Autodesk Inventor part; units mm, degrees
ref_plane "YZ Plane" through (0, 0, 0) normal (1, 0, 0) x (0, 1, 0)
ref_plane "XZ Plane" through (0, 0, 0) normal (0, 1, 0) x (-1, 0, 0)
ref_plane "XY Plane" through (0, 0, 0) normal (0, 0, 1) x (1, 0, 0)
sketch "Sketch1" plane through (0, 0, 0) normal (1, 0, 0) x (0, 1, 0)
  line L0 (0, -12) -> (3, -12)
  line L1 (3, 12) -> (0, 12)
  line L2 (0, 12) -> (0, -12)
  line L3 (3, 9) -> (3, -9)
  line L4 (3, 0) -> (0, 0)
  line L5 (0, -9.75) -> (0, 9.75)
  line L6 (3, 9.75) -> (3, -9.75)
  line L7 (3, 10.75) -> (2.15, 10.75)
  line L8 (2.15, 10.75) -> (2.15, 9.75)
  line L9 (3, 12) -> (3, 10.75)
  line L10 (2.15, 9.75) -> (3, 9.75)
  line L11 (3, -10.75) -> (2.15, -10.75)
  line L12 (2.15, -10.75) -> (2.15, -9.75)
  line L13 (2.15, -9.75) -> (3, -9.75)
  line L14 (3, -10.75) -> (3, -12)
  line L15 (0, -16.8) -> (0, 16.8)
  point P0 (1.5, 0)
  dimension "d12" = 19.5
  dimension "d13" = 1
  dimension "d14" = 0.85
  dimension "d16" = 1
revolve "Revolution1" add sketch "Sketch1" angle 360 about axis through (0, 0, -10) along (0, 0, 1)
sketch "Sketch2" plane through (0, 0, 12) normal (0, 0, 1) x (1, 0, 0)
  circle A0 centre (0, 0) radius 3
extrude "Extrusion1" cut sketch "Sketch2" against normal blind 0.25
sketch "Sketch3" plane through (0, 0, -12) normal (0, 0, -1) x (-1, 0, 0)
  circle A0 centre (0, 0) radius 3
extrude "Extrusion2" cut sketch "Sketch3" against normal blind 0.25
chamfer "Chamfer1" distance 0.5 angle 45 2 edges at (0, -3, -11.75) (0, -3, 11.75)
properties part number "hridelka1"
Part model, mm, in its own coordinate system. A direction names the side the tool comes from. Give positions to 0.01 mm unless a question says otherwise; leave off trailing zeros. Write each loop counter-clockwise with the first axis right and the second up, starting at its lowest first coordinate (ties: lowest second). Pieces come first, ordered by that corner, then holes. Notation, with made-up numbers: (-10.5, 61.5) -> (35.5, 61.5) arc R24 cw to (35.5, 81.5) -> close; hole circle Ø10 at (13.25, -37). An arc over 180 degrees is marked (long way). Put each result on its own line as item: value. Start each with the question number.
Item 1: Cut at C-C (z = 6.5). List the corners of the cut face in (x, y), then the cut area to 3 significant figures.
Item 2: Pin check, flat tips, straight feed: pin 1 Ø2 at (x, z) = (1.5, 5) entering from -Y; pin 2 Ø1.5 at (y, z) = (-2, -6.5) entering from -X; pin 3 Ø1 at (y, z) = (1.5, 4) entering from +X. Stop position of each tip, or through.
Item 3: Which spindle directions (+Z, -Z, +X, -X, +Y, -Y) get a long thin tool onto all of the face, cutting with end or side? Do faces 1 (the face through (2, 1.3, -9.75)), 2 (the face through (0, -3, -11)). Say none if no direction does.
Item 4: Cut at A-A (y = 0). List the corners of the cut face in (x, z), then the cut area to 3 significant figures.
Item 5: Pull direction Z, two halves, no side cores. Call faces 3 (the face through (0, 0, -11.75)), 4 (the face through (0, 0, 11.75)), 5 (the face through (2, 1.3, 9.75)): pulls with the +Z half, pulls with the -Z half, needs draft (parallel to the pull), parting line crosses it, or undercut.
Item 6: Wall check: L1, parallel to Z at x = 2.75, y = 0.3; L2, parallel to Y at x = 0.15, z = 0.75; L3, parallel to Y at x = 2.6, z = -1.25. Give the ranges that are in metal, low to high. Write a range as [from, to].
Answer list:
1. outline: circle Ø6 at (0, 0)
1. area: 28.3 mm2
2. pin 1: stops at y = -2.96
2. pin 2: stops at x = -2.73
2. pin 3: stops at x = 2.83
3. face 1: none
3. face 2: +Z, -Z
4. outline: (-3, -11.25) -> (-2.5, -11.75) -> (2.5, -11.75) -> (3, -11.25) -> (3, -10.75) -> (2.15, -10.75) -> (2.15, -9.75) -> (3, -9.75) -> (3, 9.75) -> (2.15, 9.75) -> (2.15, 10.75) -> (3, 10.75) -> (3, 11.25) -> (2.5, 11.75) -> (-2.5, 11.75) -> (-3, 11.25) -> (-3, 10.75) -> (-2.15, 10.75) -> (-2.15, 9.75) -> (-3, 9.75) -> (-3, -9.75) -> (-2.15, -9.75) -> (-2.15, -10.75) -> (-3, -10.75) -> close
4. area: 137 mm2
5. face 3: pulls with the -Z half
5. face 4: pulls with the +Z half
5. face 5: undercut
6. L1: z = [-11.48, -10.75], [-9.75, 9.75], [10.75, 11.48]
6. L2: y = [-3, 3]
6. L3: y = [-1.5, 1.5]
